```python
from build123d import *

# Parameters (mm, degrees)
F0_R     = 54.777634
F1_DEPTH = 25.4
F2_W     = 76.760076
F2_H     = 52.30828
F3_DEPTH = 20.32
F5_DEPTH = 12.7


with BuildPart() as f1:
    # F0 (on Front) → F1 (new body)
    with BuildSketch(Plane.XZ):
        Circle(F0_R)
    extrude(amount=F1_DEPTH)

    # F2 (on face) → F3 (cut)
    with BuildSketch(Plane.XZ.offset(25.4)):
        Rectangle(F2_W, F2_H)
    extrude(amount=-F3_DEPTH, mode=Mode.SUBTRACT)

    # F4 (on face) → F5 (join)
    with BuildSketch(Plane.XZ.offset(5.08)):
        Polygon((19.782942, 11.775956), (16.836673, 12.301875), (16.836673, -9.437174), (19.193688, -8.960415), (21.037921, -8.054476), (22.670284, -6.43198), (24.202343, -4.958846), (25.793329, -2.248279), (25.793329, 0.697988), (25.793329, 3.231779), (25.119537, 4.603426), (24.213784, 6.44728), (23.075252, 8.765006), (21.550702, 10.243896), align=None)
        Polygon((19.193688, -4.840995), (18.66336, 6.413748), (23.259537, 0.639063), align=None, mode=Mode.SUBTRACT)
        Polygon((3.131037, 12.301875), (-2.682529, -1.766953), (0, 0), (4.196519, 0), (8.598126, -8.960415), (13.575672, -8.960415), align=None)
        Polygon((5.098887, 2.528751), (1.241177, 2.483729), (3.013781, 6.77343), align=None, mode=Mode.SUBTRACT)
        Polygon((23.259537, 0.639063), (18.66336, 6.413748), (19.193688, -4.840995), align=None)
        Polygon((-27.369183, 12.301875), (-30.475451, 9.677191), (-21.320134, -8.960415), (-13.145746, 10.821605), (-16.727999, 12.301875), (-21.811419, 0), align=None)
        Polygon((-6.606236, 12.301875), (-10.039479, 12.301875), (-10.039479, -8.960415), (0, -8.960415), (0, -4.055782), (-6.606236, -4.055782), align=None)
        Polygon((3.013781, 6.77343), (1.241177, 2.483729), (5.098887, 2.528751), align=None)
    extrude(amount=F5_DEPTH)


solid = f1.part
```
CAD build for the part. Positions are in the model's coordinates, mm. A direction names the side the tool comes from. Round coordinates to 2 decimals unless told otherwise and drop trailing zeros. Write each loop counter-clockwise with the first axis right and the second up, starting at its lowest first coordinate (ties: lowest second). Pieces come first, ordered by that corner, then holes. Notation, with made-up numbers: (-16.75, 1.5) - (23.25, 1.5) arc R38 ccw to (23.25, 40.5) - close; hole circle Ø2 at (-37, -36.5). An arc over 180 degrees is marked (long way). Return JSON: item names as keys, results as strings. Group by question number.
Item 1: Band-saw the part on A-A on y = -13.25. State how many separate pieces and enclosed holes the cut face has, plus the area to 3 significant figures.
Item 2: Mould opens along X. For faces 1 (the face through (-1, -25.4, -36)), 2 (the face through (2, -11, 0)), 3 (the face through (-19.234, -11.341, 6.237)) say: +X half, -X half, draft (parallel to the pull), parting line (faces both ways), or undercut.
Item 3: 3-axis set-ups, long thin cutter, end or side, ignore diameter. For faces 4 (the face through (-1.36, -11.341, -0.896)), 5 (the face through (-1, 0, 1)): which of +Z, -Z, +X, -X, +Y, -Y reach the whole face in a straight line?
Item 4: Band-saw the part on C-C on x = 31. List the corners of the cut face in (y, z), plus the area to 3 significant figures.
Item 5: Probe probe 1 along Z at (x, y) = (22, -8.5); probe 2 along Z at (x, y) = (11, -8.5); probe 3 along Z at (x, y) = (36.5, -22.25). List the from-to ranges inside material, lowest first.
Item 6: Flat gauge pins, fed straight in: pin 1 Ø18 at (x, z) = (9.5, 5) entering from -Y; pin 2 Ø3 at (x, y) = (-26.5, -5.5) entering from +Z; pin 3 Ø4 at (x, y) = (8, -10) entering from -Z; pin 4 Ø4 at (x, z) = (-6.5, -30.5) entering from +Y. Where does each tip first touch, or does it go through?
Item 7: Band-saw the part on B-B on y = -23. List the corners of the cut face in (x, z), plus the area to 3 significant figures.
Item 8: Band-saw the part on D-D on z = 32. List the corners of the cut face in (x, y), plus the area to 3 significant figures.
Resolved:
{
 "1": {"separate pieces": "5", "enclosed holes": "1", "area": "5,910 mm²"},
 "2": {"face 1": "draft", "face 2": "undercut", "face 3": "undercut"},
 "3": {"face 4": "-Y", "face 5": "+Z, -Z, +X, -X, +Y"},
 "4": {"outline": "(-25.4, -45.16) - (0, -45.16) - (0, 45.16) - (-25.4, 45.16) - (-25.4, 26.15) - (-5.08, 26.15) - (-5.08, -26.15) - (-25.4, -26.15) - close", "area": "1,230 mm²"},
 "5": {"probe 1": "z = -50.17 to -26.15, -7.1 to 9.81, 26.15 to 50.17", "probe 2": "z = -53.66 to -26.15, -8.96 to -3.72, 26.15 to 53.66", "probe 3": "z = -40.85 to -26.15, 26.15 to 40.85"},
 "6": {"pin 1": "stops at y = -17.78", "pin 2": "stops at z = 48.74", "pin 3": "stops at z = -54.45", "pin 4": "stops at y = 0"},
 "7": {"outline": "circle Ø109.56 at (0, 0); hole (-38.38, -26.15) - (38.38, -26.15) - (38.38, 26.15) - (-38.38, 26.15) - close", "area": "5,410 mm²"},
 "8": {"outline": "(-44.46, -25.4) - (44.46, -25.4) - (44.46, 0) - (-44.46, 0) - close", "area": "2,260 mm²"}
}
